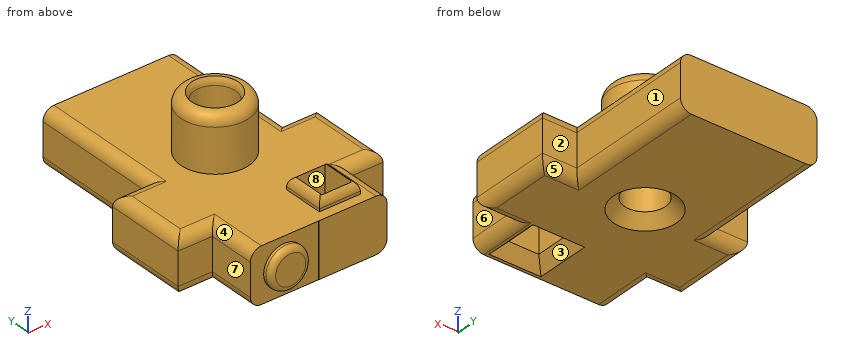
```python
from build123d import *

# Parameters (mm, degrees)
F0_W        = 19.05
F0_H        = 19.05
F0_R        = 15.875
F1_DEPTH    = 25.4
F0_R_2      = 9.525
F2_DEPTH    = 50.8
F0_W_2      = 13.97
F0_H_2      = 15.24
F3_DEPTH    = 31.75
F4_R        = 9.525
F5_DEPTH    = 3.81
F6_R        = 2.54
F7_R        = 5.08
F9_T1_DEPTH = 44.45
F9_T3_DEPTH = 44.45
F10_R       = 5.08
F11_SIZE    = 5.08
F12_SIZE    = 5.08


# Not quite as in the source:
# - a fillet or chamfer that OpenCascade refuses, or shapes differently, is made with other operations: its cross-section is extruded or revolved along the edge and cut away or added


with BuildPart() as f1:
    # F0 (on Top) → F1 (new body)
    with BuildSketch(Plane.XY):
        Polygon((31.75, 60.325), (0, 60.325), (-31.75, 60.325), (-31.75, 0), (-47.625, 0), (-47.625, -38.1), (-31.75, -38.1), (-31.75, -60.325), (0, -60.325), (0, -60.3444650769), (31.75, -60.3444650769), (31.75, -38.1), (47.7005839348, -38.1), (47.7005839348, 0), (47.625, 0), (31.75, 0), align=None)
        with Locations((13.5087583899, -46.2022918522)):
            Rectangle(F0_W, F0_H, mode=Mode.SUBTRACT)
        Circle(F0_R, mode=Mode.SUBTRACT)
    extrude(amount=F1_DEPTH)

    # F0 (on Top) → F2 (join)
    with BuildSketch(Plane.XY):
        Circle(F0_R)
        Circle(F0_R_2, mode=Mode.SUBTRACT)
    extrude(amount=F2_DEPTH)

    # F0 (on Top) → F3 (join)
    with BuildSketch(Plane.XY):
        with Locations((13.5087583899, -46.2022918522)):
            Rectangle(F0_W, F0_H)
        with Locations((13.3824522054, -46.1642474878)):
            Rectangle(F0_W_2, F0_H_2, mode=Mode.SUBTRACT)
    extrude(amount=F3_DEPTH)

    # F4 (on face) → F5 (join)
    with BuildSketch(Plane.XZ.offset(60.325)):
        with Locations((-16.0763879821, 12.6689534055)):
            Circle(F4_R)
    extrude(amount=F5_DEPTH)

    # F6
    f6_edges = [f1.edges().sort_by_distance(p)[0] for p in [
        (-25.601388, -64.135, 12.668953),
    ]]
    fillet(f6_edges, radius=F6_R)

    # F7
    f7_edges = [f1.edges().sort_by_distance(p)[0] for p in [
        (-15.875, 0, 50.8),
    ]]
    fillet(f7_edges, radius=F7_R)

    # F8: fillet of radius 5.08 on 1 edges, made by hand

    # F8_s1 → F8_t2 (revolve, cut)
    with BuildSketch(Plane.XZ):
        with BuildLine():
            ThreePointArc((10.795, 50.8), (9.8530951188, 49.2359470592), (9.525, 47.4398958349))
            Line((9.525, 47.4398958349), (9.525, 50.8))
            Line((9.525, 50.8), (10.795, 50.8))
        make_face()
    revolve(axis=Axis((0, 0, 50.8), (0, 0, 1)), mode=Mode.SUBTRACT)

    # F9: fillet of radius 5.08 on 4 edges, made by hand

    # F9_s2 → F9_t1 (cut)
    with BuildSketch(Plane.XZ.offset(23.9772918522)):
        with BuildLine():
            ThreePointArc((3.9837583899, 26.67), (5.4716559415, 30.2621024484), (9.0637583899, 31.75))
            Line((9.0637583899, 31.75), (3.9837583899, 31.75))
            Line((3.9837583899, 31.75), (3.9837583899, 26.67))
        make_face()
        with BuildLine():
            ThreePointArc((23.0337583899, 26.67), (21.5458608384, 30.2621024484), (17.9537583899, 31.75))
            Line((17.9537583899, 31.75), (23.0337583899, 31.75))
            Line((23.0337583899, 31.75), (23.0337583899, 26.67))
        make_face()
    extrude(amount=F9_T1_DEPTH, mode=Mode.SUBTRACT)

    # F9_s4 → F9_t3 (cut)
    with BuildSketch(Plane.YZ.offset(-8.7162416101)):
        with BuildLine():
            ThreePointArc((-36.6772918522, 26.67), (-38.1651894038, 30.2621024484), (-41.7572918522, 31.75))
            Line((-41.7572918522, 31.75), (-36.6772918522, 31.75))
            Line((-36.6772918522, 31.75), (-36.6772918522, 26.67))
        make_face()
        with BuildLine():
            ThreePointArc((-55.7272918522, 26.67), (-54.2393943007, 30.2621024484), (-50.6472918522, 31.75))
            Line((-50.6472918522, 31.75), (-55.7272918522, 31.75))
            Line((-55.7272918522, 31.75), (-55.7272918522, 26.67))
        make_face()
    extrude(amount=F9_T3_DEPTH, mode=Mode.SUBTRACT)

    # F10
    f10_edges = [f1.edges().sort_by_distance(p)[0] for p in [
        (39.725292, -38.1, 25.4),
        (31.75, -49.222233, 25.4),
        (-31.75, -49.2125, 25.4),
        (-39.6875, -38.1, 25.4),
        (-31.75, 30.1625, 25.4),
        (-39.6875, 0, 25.4),
        (39.725292, 0, 25.4),
        (31.75, 30.1625, 25.4),
        (-31.75, -49.2125, 0),
        (-31.75, 30.1625, 0),
        (-39.6875, 0, 0),
        (-39.6875, -38.1, 0),
        (-47.625, -19.05, 0),
        (31.75, 30.1625, 0),
        (31.75, -49.222233, 0),
        (39.725292, -38.1, 0),
        (47.700584, -19.05, 0),
        (39.725292, 0, 0),
        (47.700584, -19.05, 25.4),
        (-47.625, -19.05, 25.4),
    ]]
    fillet(f10_edges, radius=F10_R)

    # F11
    f11_edges = [f1.edges().sort_by_distance(p)[0] for p in [
        (13.382452, -38.544247, 0),
        (20.367452, -46.164247, 0),
        (13.382452, -53.784247, 0),
        (6.397452, -46.164247, 0),
    ]]
    chamfer(f11_edges, length=F11_SIZE)

    # F12
    f12_edges = [f1.edges().sort_by_distance(p)[0] for p in [
        (-9.525, 0, 0),
    ]]
    chamfer(f12_edges, length=F12_SIZE)


solid = f1.part
```
CAD build for the part. Positions are in the model's coordinates, mm. Face numbers are marked on the shaded views. A direction names the side the tool comes from. Round coordinates to 2 decimals unless told otherwise and drop trailing zeros. Write each loop counter-clockwise with the first axis right and the second up, starting at its lowest first coordinate (ties: lowest second). Pieces come first, ordered by that corner, then holes.
Item 1: Band-saw the part on B-B on x = 40.5. Write the cut outline in (y, z), then the cut area to 3 significant figures.
Filled in:
outline: (-38.1, 5.08) arc R5.08 ccw to (-33.02, 0) - (-5.08, 0) arc R5.08 ccw to (0, 5.08) - (0, 20.32) arc R5.08 ccw to (-5.08, 25.4) - (-33.02, 25.4) arc R5.08 ccw to (-38.1, 20.32) - close
area: 946 mm2
Item 2: Band-saw the part on C-C on y = 19. Write the cut outline in (x, z), then the cut area to 3 significant figures.
Filled in:
outline: (-31.75, 5.08) arc R5.08 ccw to (-26.67, 0) - (26.67, 0) arc R5.08 ccw to (31.75, 5.08) - (31.75, 20.32) arc R5.08 ccw to (26.67, 25.4) - (-26.67, 25.4) arc R5.08 ccw to (-31.75, 20.32) - close
area: 1,590 mm2
Item 3: Tool access for the marked faces 4, 5, 6, 7 and 8: list every direction of +Z, -Z, +X, -X, +Y, -Y with a clear straight run to the whole face (end or side of a thin tool).
Filled in:
face 4: +Z, -X, -Y
face 5: -Z, +X, +Y
face 6: +Z, -Z, +X, -Y
face 7: +Z, -Z, -X, -Y
face 8: +Z, -Z
Item 4: Drop flat-ended pins along their axis: pin 1 Ø12 at (x, z) = (-36, 11) entering from -Y (3 decimals); pin 2 Ø12 at (y, z) = (25, 29.5) entering from +X; pin 3 Ø5 at (x, y) = (-18.5, 12) entering from +Z. Give the stop position or say it passes through.
Filled in:
pin 1: stops at y = -60.325
pin 2: stops at x = 30.63
pin 3: stops at z = 25.4
Item 5: Drill centre lines: L1, parallel to Y at x = 0, z = 32 (3 decimals); L2, parallel to Y at x = 0, z = 14.5 (3 decimals); L3, parallel to X at y = -55, z = 9. Where is each one in solid material? Low to high.
Filled in:
L1: y = -15.875 to -9.525, 9.525 to 15.875
L2: y = -60.325 to -9.525, 9.525 to 60.325
L3: x = -31.75 to 31.75
Item 6: Band-saw the part on A-A on y = -51.5. Write the cut outline in (x, z).
Filled in:
outline: (-31.75, 5.08) arc R5.08 ccw to (-26.67, 0) - (1.32, 0) - (6.4, 5.08) - (6.4, 30.99) arc R5.08 ccw to (3.98, 26.67) - (3.98, 25.4) - (-26.67, 25.4) arc R5.08 ccw to (-31.75, 20.32) - close; (20.37, 5.08) - (25.45, 0) - (26.67, 0) arc R5.08 ccw to (31.75, 5.08) - (31.75, 20.32) arc R5.08 ccw to (26.67, 25.4) - (23.03, 25.4) - (23.03, 26.67) arc R5.08 ccw to (20.37, 31.14) - close
Item 7: Mould opens along X. For the marked faces 1, 2 and 3 say: released by +X, released by -X, zero draft, split by the parting line, or undercut.
Filled in:
face 1: released by +X
face 2: zero draft
face 3: undercut
